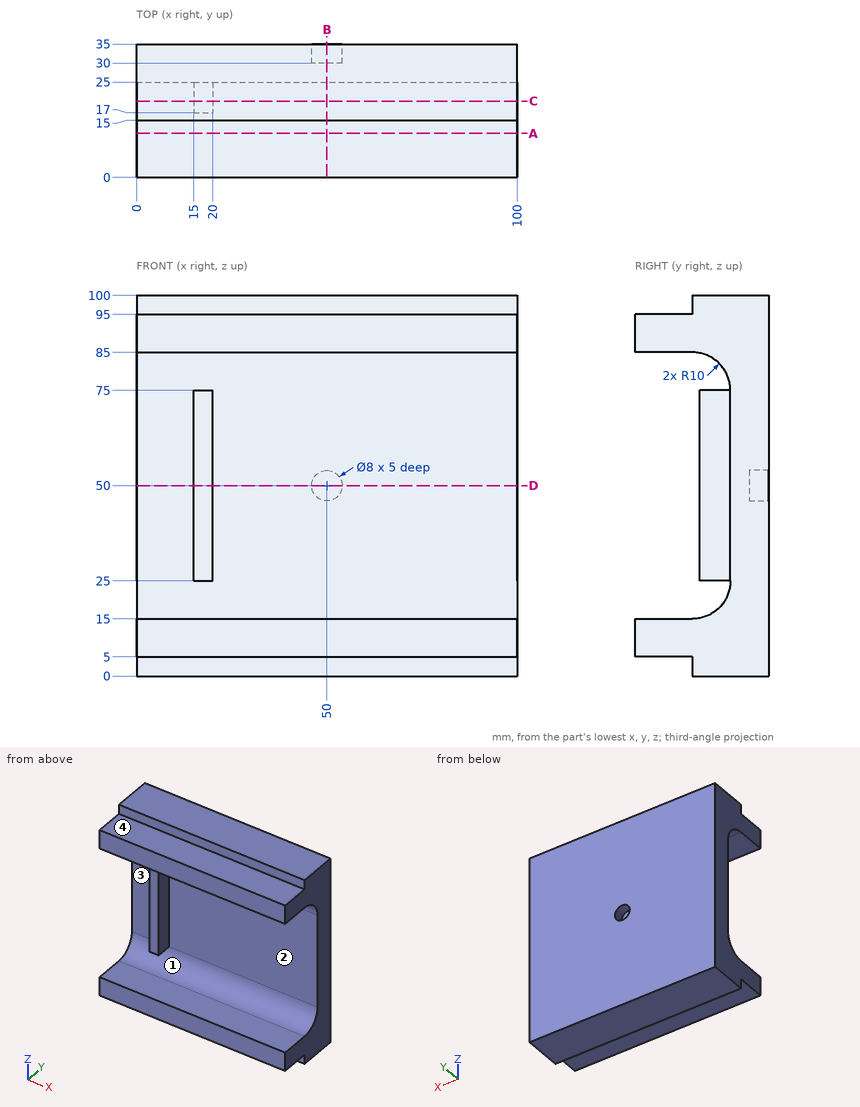
Drawing for the job (mm, zero at the part's lowest x, y, z). A direction names the side the tool comes from. Round coordinates to 2 decimals unless told otherwise and drop trailing zeros. Write each loop counter-clockwise with the first axis right and the second up, starting at its lowest first coordinate (ties: lowest second). Pieces come first, ordered by that corner, then holes. Notation, with made-up numbers: M 78.25,-2 L 94.25,-2 A28 cw 94.25,23 Z; hole C 41,30 d7. An arc over 180 degrees is marked long. Answer in a Markdown table with one row per item.
1. Probe L1, parallel to Z at x = 16, y = 2; L2, parallel to X at y = 33.7, z = 50; L3, parallel to Y at x = 82, z = 62. List the from-to ranges inside material, lowest first. Write a range as [from, to].
Geometry check:
| item | result |
|---|---|
| L1 | [5, 15], [85, 95] |
| L2 | [0, 46], [54, 100] |
| L3 | [25, 35] |
2. Which spindle directions (+Z, -Z, +X, -X, +Y, -Y) get a long thin tool onto all of the face, cutting with end or side? Do the marked faces 1, 2, 3 and 4. Say none if no direction does.
Geometry check:
| item | result |
|---|---|
| face 1 | +X, -X, -Y |
| face 2 | +X, -Y |
| face 3 | -X, -Y |
| face 4 | +Z, +X, -X, -Y |
3. Flat gauge pins, fed straight in: P1, Ø7.5, axis at x = 10, z = 58.5, coming from the -Y side; P2, Ø5.5, axis at x = 39.5, z = 2, coming from the -Y side; P3, Ø1.5, axis at x = 18, z = 39.5, coming from the -Y side; P4, Ø3, axis at x = 60, y = 30.5, coming from the -Z side. Where does each tip first touch, or does it go through?
Geometry check:
| item | result |
|---|---|
| P1 | y = 25 |
| P2 | y = 15 |
| P3 | y = 17 |
| P4 | z = 0 |
4. Saw through at D-D (z = 50). List the corners of the cut face in (x, y), and give its area (3 significant figures).
Geometry check:
| item | result |
|---|---|
| outline | M 0,25 L 15,25 L 15,17 L 20,17 L 20,25 L 100,25 L 100,35 L 54,35 L 54,30 L 46,30 L 46,35 L 0,35 Z |
| area | 1,000 mm2 |
5. Saw through at C-C (y = 20). List the corners of the cut face in (x, z).
Geometry check:
| item | result |
|---|---|
| outline | M 0,0 L 100,0 L 100,16.34 L 0,16.34 Z; M 0,83.66 L 100,83.66 L 100,100 L 0,100 Z; M 15,25 L 20,25 L 20,75 L 15,75 Z |
6. Saw through at B-B (x = 50). List the corners of the cut face in (y, z), and give its area (3 significant figures).
Geometry check:
| item | result |
|---|---|
| outline | M 0,5 L 15,5 L 15,0 L 35,0 L 35,46 L 30,46 L 30,54 L 35,54 L 35,100 L 15,100 L 15,95 L 0,95 L 0,85 L 15,85 A10 cw 25,75 L 25,25 A10 cw 15,15 L 0,15 Z |
| area | 1,600 mm2 |
7. Saw through at A-A (y = 11.5). List the corners of the cut face in (x, z).
Geometry check:
| item | result |
|---|---|
| outline | M 0,5 L 100,5 L 100,15 L 0,15 Z; M 0,85 L 100,85 L 100,95 L 0,95 Z |
